Source: CAD feature listing. Evaluate the final solid. Frame: model axes, mm. Coordinates: 2 decimals unless noted, no trailing zeros. Write each loop counter-clockwise with the first axis right and the second up, starting at its lowest first coordinate (ties: lowest second). Pieces come first, ordered by that corner, then holes. Notation, with made-up numbers: (-21, -31.75) -> (9, -31.75) arc R17 cw to (9, -24.75) -> close; hole circle Ø11 at (-14, -5). An arc over 180 degrees is marked (long way). Write item = value, one per line.
Autodesk Inventor part; units mm, degrees
ref_plane "YZ Plane" through (0, 0, 0) normal (1, 0, 0) x (0, 1, 0)
ref_plane "XZ Plane" through (0, 0, 0) normal (0, 1, 0) x (-1, 0, 0)
ref_plane "XY Plane" through (0, 0, 0) normal (0, 0, 1) x (1, 0, 0)
sketch "Sketch1" plane through (0, 0, 0) normal (0, 1, 0) x (-1, 0, 0)
  line L0 (0, 0) -> (250, 0)
  line L1 (0, -140) -> (0, 0)
  line L2 (250, 0) -> (250, -70)
  line L3 (250, 0) -> (125, 0)
  line L4 (125, 0) -> (125, -70)
  line L5 (125, -70) -> (250, -70)
  line L6 (250, -70) -> (250, 0)
  line L7 (250, 0) -> (220, 0)
  line L8 (220, 0) -> (220, -30)
  line L9 (220, -30) -> (150, -30)
  line L10 (150, -30) -> (150, 0)
  line L11 (250, 0) -> (247, 0)
  line L12 (247, 0) -> (247, -20)
  line L13 (247, -20) -> (250, -20)
  line L14 (247, -20) -> (247, -70)
  line L15 (250, -20) -> (250, -40)
  line L16 (250, -40) -> (250, -60)
  line L17 (250, -60) -> (247, -60)
  line L18 (250, -40) -> (247, -40)
  dimension "d2" = 125
  dimension "d3" = 70
  dimension "d5" = 30
  dimension "d6" = 70
  dimension "d7" = 3
  dimension "d8" = 20
  dimension "d9" = 20
  dimension "d10" = 20
extrude "Extrusion1" add sketch "Sketch1" along normal blind 3 contours L0 L10 L9 L8 L12 L14 L5 L4 | L0 L2 L13 L12 | L14 L18 L2 L17
mirror "Mirror1" about plane through (-125, 0, -70) normal (0, 0, -1) of "Extrusion1"
mirror "Mirror2" about plane through (-125, 0, 0) normal (1, 0, 0) of "Extrusion1", "Mirror1"
properties part number "onderkant"
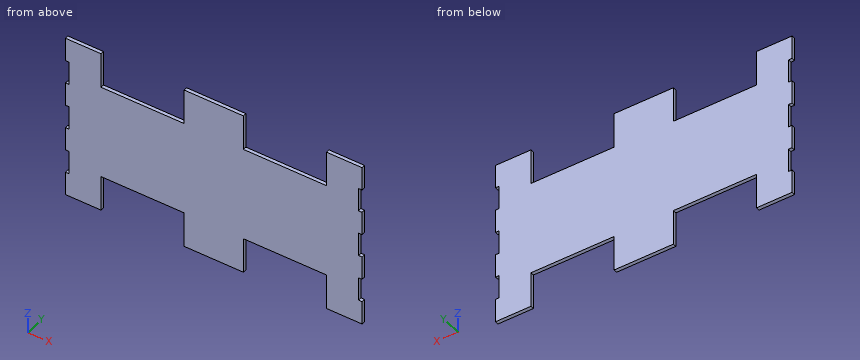
1) First-contact query: pin 1 Ø1.5 at (x, y) = (-93.5, 2.5) entering from -Z; pin 2 Ø1.5 at (y, z) = (2, -20.5) entering from +X. Flat tips, straight axial feed; report the tip coordinate or a pass-through.
Answer block:
pin_1 = -110
pin_2 = 0
2) Cut plane A-A, the plane x = -168.5. Output: boundary loops of the cut face in (y, z).
Answer block:
outline = (0, -110) -> (3, -110) -> (3, -30) -> (0, -30) -> close
3) Material intervals for probe 1 along X at (y, z) = (0.3, -128); probe 2 along X at (y, z) = (2.25, -111); probe 3 along Z at (x, y) = (-86, 2.7), sorted ascending. Write a range as [from, to].
Answer block:
probe_1 = [-250, -220], [-150, -100], [-30, 0]
probe_2 = [-247, -220], [-150, -100], [-30, -3]
probe_3 = [-110, -30]
4) Cut plane B-B, the plane z = -75. Output: boundary loops of the cut face in (x, y), and give its area (3 significant figures).
Answer block:
outline = (-247, 0) -> (-3, 0) -> (-3, 3) -> (-247, 3) -> close
area = 732 mm2
